Input: dimensioned drawing with shaded views. Units: mm. Origin: part minimum x, y, z. A direction names the side the tool comes from. Coordinates: 2 decimals unless noted, no trailing zeros. Order: outer loops, then holes, each group sorted by start corner. A loop starts at its lowest first (then second) coordinate and runs counter-clockwise, first axis right, second up. Notation, with made-up numbers: (-39.5, -20.5) - (7.5, -20.5) arc R21 ccw to (7.5, -5.5) - close; hole circle Ø6 at (-32, -12.5). An arc over 180 degrees is marked (long way). One line per question, with ' | ' between items. Start each with the question number.
(1) Section A-A (y = 25.4). Return the cut outline in (x, z) (3 decimals).
(2) Access query for the marked faces 5, 6, 7 and 8. Directions: +Z, -Z, +X, -X, +Y, -Y. A direction counts if a zero-diameter tool reaches every point of the face in a straight line with its end or side. Return the directions, or none.
(3) Line query: line 1 along X through (y, z) = (2, 21); line 2 along Y through (x, z) = (42, 25); line 3 along Z through (x, y) = (28.5, 26). Output: solid intervals per line, ascending.
(4) Contact query for flat-ended pins moving along their axis: P1, Ø2, axis at x = 39.5, y = 12.5, coming from the -Z side; P2, Ø10, axis at x = 68.5, y = 6.5, coming from the +Z side (3 decimals); P3, Ø4, axis at x = 20.5, y = 15.5, coming from the +Z side. Output: stop coordinate, or through.
(5) Draft query along X for the marked faces 1, 2, 3 and 4. Return one class per face: +X half, -X half, draft (parallel to the pull), parting line (faces both ways), or undercut.
(6) Section D-D (y = 8.5). Return the cut outline in (x, z) (1 decimal).
(7) Section C-C (z = 43). Return the cut outline in (x, y), then the cut area to 3 significant figures.
(8) Section B-B (x = 61.5). Return the cut outline in (y, z) (1 decimal).
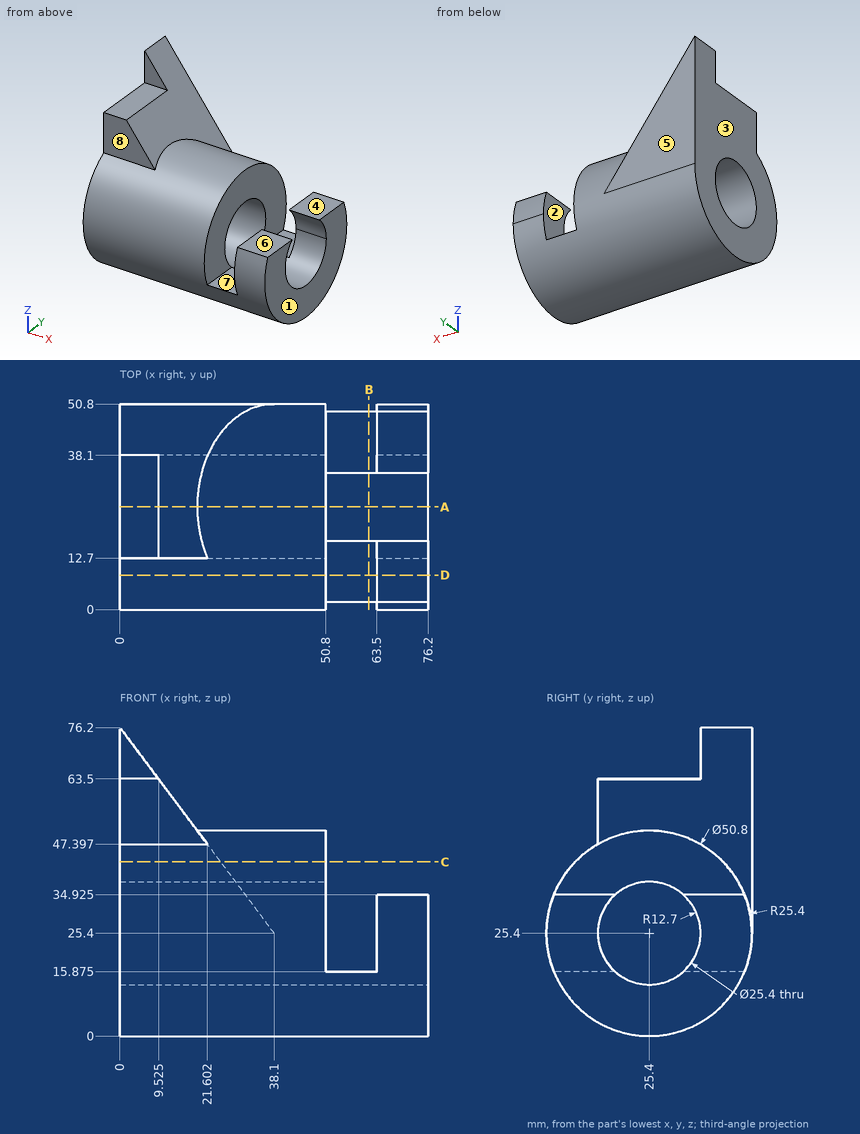
Response values:
1) outline: (0, 0) - (76.2, 0) - (76.2, 12.7) - (0, 12.7) - close; (0, 38.1) - (50.8, 38.1) - (50.8, 50.8) - (19.05, 50.8) - (9.525, 63.5) - (0, 63.5) - close
2) face 5: +Z, -Z, +X, -X, +Y | face 6: +Z, +X, +Y, -Y | face 7: +Z, +Y, -Y | face 8: +Z, +X, -X, -Y
3) line 1: x = 0 to 50.8, 63.5 to 76.2 | line 2: y = 0 to 12.71, 38.09 to 50.8 | line 3: z = 0.01 to 12.71, 38.09 to 50.79
4) P1: stops at z = 2.96 | P2: stops at z = 34.925 | P3: stops at z = 51.53
5) face 1: +X half | face 2: undercut | face 3: -X half | face 4: draft
6) outline: (0, 6.4) - (76.2, 6.4) - (76.2, 34.9) - (63.5, 34.9) - (63.5, 15.9) - (50.8, 15.9) - (50.8, 44.4) - (0, 44.4) - close
7) outline: (0, 7.09) - (50.8, 7.09) - (50.8, 43.71) - (24.9, 43.71) - (24.9, 50.8) - (0, 50.8) - close | area: 2,040 mm²
8) outline: (1.9, 15.9) arc R25.4 ccw to (48.9, 15.9) - (33.8, 15.9) arc R12.7 cw to (17, 15.9) - close
